from build123d import *

# Parameters (mm, degrees)
F1_DEPTH = 89.154
F2_DEPTH = 131.064
F3_R     = 11.0199394835
F4_DEPTH = 25.4
F3_R_2   = 11.0346787259
F5_DEPTH = 138.938


with BuildPart() as f1:
    # F0 (on Front) → F1 (new body, symmetric)
    with BuildSketch(Plane.XZ):
        with BuildLine():
            Line((-73.9898234606, 53.6717362702), (-69.6088522673, -60.0099079311))
            Line((-69.6088522673, -60.0099079311), (63.2807761431, -60.0099079311))
            Line((63.2807761431, -60.0099079311), (63.2807761431, 53.6717362702))
            Line((63.2807761431, 53.6717362702), (46.2222844362, 53.6717362702))
            ThreePointArc((46.2222844362, 53.6717362702), (-7.294902578, 4.3339080113), (-60.8120895922, 53.6717362702))
            Line((-60.8120895922, 53.6717362702), (-73.9898234606, 53.6717362702))
        make_face()
        with BuildLine():
            Line((-46.6877035797, 53.6717362702), (-60.8120895922, 53.6717362702))
            ThreePointArc((-60.8120895922, 53.6717362702), (-7.294902578, 4.3339080113), (46.2222844362, 53.6717362702))
            Line((46.2222844362, 53.6717362702), (24.9031372368, 53.6717362702))
            ThreePointArc((24.9031372368, 53.6717362702), (-10.8922831714, 18.0866857546), (-46.6877035797, 53.6717362702))
        make_face()
    extrude(amount=F1_DEPTH, both=True)

    # F0 (on Front) → F2 (join, symmetric)
    with BuildSketch(Plane.XZ):
        with BuildLine():
            Line((-46.6877035797, 53.6717362702), (-60.8120895922, 53.6717362702))
            ThreePointArc((-60.8120895922, 53.6717362702), (-7.294902578, 4.3339080113), (46.2222844362, 53.6717362702))
            Line((46.2222844362, 53.6717362702), (24.9031372368, 53.6717362702))
            ThreePointArc((24.9031372368, 53.6717362702), (-10.8922831714, 18.0866857546), (-46.6877035797, 53.6717362702))
        make_face()
    extrude(amount=F2_DEPTH, both=True)


with BuildPart() as f4:
    # F3 (on Top) → F4 (new body)
    with BuildSketch(Plane.XY):
        with Locations((39.523396641, 44.7258390486)):
            Circle(F3_R)
    extrude(amount=F4_DEPTH)


with BuildPart() as f4b:
    # F3 (on Top) → F4, piece 2 (new body)
    with BuildSketch(Plane.XY):
        with Locations((-60.1624064147, 30.0455577672)):
            Circle(F3_R_2)
    extrude(amount=F4_DEPTH)


with BuildPart() as f5_tool:
    # F3 (on Top) → F5 (new body, symmetric)
    with BuildSketch(Plane.XY):
        with Locations((39.523396641, 44.7258390486)):
            Circle(F3_R)
        with Locations((-60.1624064147, 30.0455577672)):
            Circle(F3_R_2)
    extrude(amount=F5_DEPTH, both=True)


with BuildPart() as f1_1:
    add(f1.part)

    # F5: cut by f5_tool
    add(f5_tool.part, mode=Mode.SUBTRACT)


with BuildPart() as f4_1:
    add(f4.part)

    # F5: cut by f5_tool
    add(f5_tool.part, mode=Mode.SUBTRACT)


with BuildPart() as f4b_1:
    add(f4b.part)

    # F5: cut by f5_tool
    add(f5_tool.part, mode=Mode.SUBTRACT)


solid = f1_1.part
Could you check a few things on this model? Use its own coordinates, in mm. A direction names the side the tool comes from. Coordinates: 2 decimals unless noted, no trailing zeros. Order: outer loops, then holes, each group sorted by start corner. A loop starts at its lowest first (then second) coordinate and runs counter-clockwise, first axis right, second up. Notation, with made-up numbers: (47, 55) -> (75, 55) arc R15 cw to (75, 65) -> close; hole circle Ø7 at (74, 17). An arc over 180 degrees is marked (long way). One line per item, written item: value. Start each with the question number.
1) I'm going to push flat-ended pins straight in: pin 1 (6 mm diameter, centred on x = 49, z = -10.5, fed in from -Y); pin 2 (5 mm diameter, centred on x = -31.5, y = -101, fed in from +Z); pin 3 (12 mm diameter, centred on x = 28, z = -36.5, fed in from +Y); pin 4 (17.5 mm diameter, centred on x = 39.52, y = 44.73, fed in from -Z). Where does each tip first touch, or does it pass through?
2) Imagine slicing it at A-A on z = 40. List the corners of the cut face in (x, y) for me.
3) Imagine slicing it at D-D on y = -81. List the corners of the cut face in (x, z) for me, plus the area to 3 significant figures.
4) Imagine slicing it at C-C on z = -50. List the corners of the cut face in (x, y) for me, plus the area to 3 significant figures.
5) We'd pull the mould along X, two halves only. Please class faces 1 (the cylindrical face through (-49.637, 33.36, -2.373)), 2 (the cylindrical face through (-8.415, -110.402, 4.346)), 3 (the flat face through (4, 131.064, 18)): +X half, -X half, draft (parallel to the pull), parting line (faces both ways), or undercut.
6) Imagine slicing it at B-B on x = 39. List the corners of the cut face in (y, z) for me, plus the area to 3 significant figures.
7) If I drill on L1, parallel to Y at x = -59.5, z = 34; L2, parallel to X at y = 23, z = 45.5 (3 decimals); L3, parallel to Y at x = -7, z = -43, over which ranges is the centre line in solid material (lowest first)? Write a range as [from, to].
8) Which directions (+Z, -Z, +X, -X, +Y, -Y) give clear straight access to the entire face, cutting with the end or side of a thin tool? Please do faces 4 (the flat face through (44, -2, 53.672)), 5 (the cylindrical face through (-8.415, 109.816, 4.346)).
Answer list:
1. pin 1: stops at y = -89.15
1. pin 2: stops at z = 26.54
1. pin 3: stops at y = 89.15
1. pin 4: passes through
2. outline: (-73.46, -89.15) -> (-57.87, -89.15) -> (-57.87, -131.06) -> (-43.89, -131.06) -> (-43.89, 131.06) -> (-57.87, 131.06) -> (-57.87, 89.15) -> (-73.46, 89.15) -> close; (22.1, -131.06) -> (43.28, -131.06) -> (43.28, -89.15) -> (63.28, -89.15) -> (63.28, 89.15) -> (43.28, 89.15) -> (43.28, 131.06) -> (22.1, 131.06) -> close; hole circle Ø22.07 at (-60.16, 30.05); hole circle Ø22.04 at (39.52, 44.73)
3. outline: (-73.99, 53.67) -> (-69.61, -60.01) -> (63.28, -60.01) -> (63.28, 53.67) -> (24.9, 53.67) arc R35.8 cw to (-46.69, 53.67) -> close
3. area: 13,400 mm2
4. outline: (-69.99, -89.15) -> (63.28, -89.15) -> (63.28, 89.15) -> (-69.99, 89.15) -> (-69.99, 35.05) arc R11.03 cw (long way) to (-69.99, 25.04) -> close; hole circle Ø22.04 at (39.52, 44.73)
4. area: 23,000 mm2
5. face 1: undercut
5. face 2: parting line
5. face 3: draft
6. outline: (-131.06, 30.83) -> (-89.15, 30.83) -> (-89.15, -60.01) -> (33.72, -60.01) -> (33.72, 53.67) -> (-131.06, 53.67) -> close; (55.73, -60.01) -> (89.15, -60.01) -> (89.15, 30.83) -> (131.06, 30.83) -> (131.06, 53.67) -> (55.73, 53.67) -> close
6. area: 19,700 mm2
7. L1: y = [-89.15, 19.03], [41.06, 89.15]
7. L2: x = [-73.675, -68.655], [-51.67, -45.693], [23.908, 63.281]
7. L3: y = [-89.15, 89.15]
8. face 4: +Z, +X, -X, +Y, -Y
8. face 5: -Z, +Y
